```python
from build123d import *

# Parameters (mm, degrees)
SKETCH_1_R           = 3.5
EXTRUDE_1_DEPTH      = 3
SKETCH_2_R           = 1.5
CUT_EXTRUDE_1_DEPTH  = 10
EXTRUDE_2_DEPTH      = 4
EXTRUDE_5_DEPTH      = 7
FILLET_1_R           = 2
HOLE_WIZARD_M2_5_1_D = 2.05
SKETCH_12_R          = 1.025
EXTRUDE_6_DEPTH      = 5
EXTRUDE_7_DEPTH      = 2.5
CUT_EXTRUDE_START    = 2.5
SKETCH_14_W          = 65.294749478
SKETCH_14_H          = 102.548808998
CUT_EXTRUDE_2_DEPTH  = 93.634928881
CUT_EXTRUDE_3_DEPTH  = 2.5
SKETCH_16_R          = 1.35
CUT_EXTRUDE_4_DEPTH  = 10
EXTRUDE_START        = 1
SKETCH_17_R          = 1.35
EXTRUDE_8_DEPTH      = 1
FILLET_2_R           = 3


with BuildPart() as part:
    # 草图1 → 凸台-拉伸1 (new body)
    with BuildSketch(Plane.XY):
        with BuildLine():
            Line((0, 0), (17, 0))
            Line((17, 0), (17, 21))
            ThreePointArc((17, 21), (14.559389791, 26.961023013), (8.639106973, 29.498861644))
            ThreePointArc((8.639106973, 29.498861644), (4.214678609, 30.921411086), (1.327625741, 34.563407653))
            ThreePointArc((1.327625741, 34.563407653), (-5.234705957, 62.223549547), (-3.748501306, 90.612611571))
            ThreePointArc((-3.748501306, 90.612611571), (-5.162788524, 92.923505905), (-7.58241645, 91.704554856))
            ThreePointArc((-7.58241645, 91.704554856), (-12.196269834, 55.45091149), (0, 21))
            Line((0, 21), (0, 0))
        make_face()
        with Locations((8.5, 21)):
            Circle(SKETCH_1_R, mode=Mode.SUBTRACT)
    extrude(amount=EXTRUDE_1_DEPTH)

    # 草图2 → 切除-拉伸1 (cut)
    with BuildSketch(Plane(origin=(0, 0, 0), x_dir=(-1, 0, 0), z_dir=(0, 0, -1))):
        with Locations((-14, 4)):
            Circle(SKETCH_2_R)
        with Locations(Location((-3, 4, 0), (0, 0, 180))):
            Circle(SKETCH_2_R)
    extrude(amount=-CUT_EXTRUDE_1_DEPTH, mode=Mode.SUBTRACT)

    # 草图3 → 凸台-拉伸2 (add)
    with BuildSketch(Plane.XY.offset(3)):
        with BuildLine():
            ThreePointArc((-7.58241645, 91.704554856), (-12.6426678, 63.080202535), (-7.007767698, 34.563407653))
            Line((-7.007767698, 34.563407653), (1.327625741, 34.563407653))
            ThreePointArc((1.327625741, 34.563407653), (-5.234705957, 62.223549547), (-3.748501306, 90.612611571))
            ThreePointArc((-3.748501306, 90.612611571), (-5.162788524, 92.923505905), (-7.58241645, 91.704554856))
        make_face()
    extrude(amount=EXTRUDE_2_DEPTH)

    # 草图8 → 凸台-拉伸5 (add)
    with BuildSketch(Plane(origin=(0, 0, 0), x_dir=(-1, 0, 0), z_dir=(0, 0, -1))):
        with BuildLine():
            Line((8.353336216, 89.563407653), (13.622203114, 89.563407653))
            ThreePointArc((13.622203114, 89.563407653), (17.624786926, 61.957713987), (12.366747323, 34.563407653))
            Line((12.366747323, 34.563407653), (7.007767698, 34.563407653))
            ThreePointArc((7.007767698, 34.563407653), (12.623031035, 61.942490485), (8.353336216, 89.563407653))
        make_face()
    extrude(amount=-EXTRUDE_5_DEPTH)

    # 圆角1
    fillet_1_edges = [part.edges().sort_by_distance(p)[0] for p in [
        (-12.366747323, 34.563407653, 3.5),
        (-13.622203114, 89.563407653, 3.5),
        (-8.353336216, 89.563407653, 3.5),
        (-7.007767698, 34.563407653, 1.5),
    ]]
    fillet(fillet_1_edges, radius=FILLET_1_R)

    # M2.5 螺纹孔1 (through all)
    with Locations(Plane(origin=(0, 0, 0), x_dir=(-1, 0, 0), z_dir=(0, 0, -1))):
        with Locations((14.33753876, 52.418963936), (-20.3596947, 65.689324708), (13.008857265, 82.418963936), (15.069556912, 67.418963936)):
            Hole(HOLE_WIZARD_M2_5_1_D / 2)

    # 草图12 → 凸台-拉伸6 (add)
    with BuildSketch(Plane(origin=(0, 0, 0), x_dir=(-1, 0, 0), z_dir=(0, 0, -1))):
        with BuildLine():
            Line((7.545930127, 34.563407653), (8.350121818, 34.563407653))
            Line((8.350121818, 34.563407653), (10.964814809, 34.563407653))
            ThreePointArc((10.964814809, 34.563407653), (12.119748759, 34.930579564), (12.850623405, 35.897280083))
            ThreePointArc((12.850623405, 35.897280083), (17.623972952, 61.922380585), (14.065160369, 88.141182522))
            ThreePointArc((14.065160369, 88.141182522), (13.343005034, 89.168952691), (12.150434226, 89.563407653))
            Line((12.150434226, 89.563407653), (9.767172344, 89.563407653))
            Line((9.767172344, 89.563407653), (8.88187432, 89.563407653))
            ThreePointArc((8.88187432, 89.563407653), (13.123220294, 61.944160836), (7.545930127, 34.563407653))
        make_face()
        with Locations((14.33753876, 52.418963936)):
            Circle(SKETCH_12_R, mode=Mode.SUBTRACT)
        with Locations((15.069556912, 67.418963936)):
            Circle(SKETCH_12_R, mode=Mode.SUBTRACT)
        with Locations((13.008857265, 82.418963936)):
            Circle(SKETCH_12_R, mode=Mode.SUBTRACT)
    extrude(amount=EXTRUDE_6_DEPTH)

    # 草图13 → 凸台-拉伸7 (add)
    with BuildSketch(Plane(origin=(0, 0, -5), x_dir=(-1, 0, 0), z_dir=(0, 0, -1))):
        with BuildLine():
            Line((-1.327625741, 34.563407653), (7.545930127, 34.563407653))
            ThreePointArc((7.545930127, 34.563407653), (13.123220294, 61.944160836), (8.88187432, 89.563407653))
            Line((8.88187432, 89.563407653), (3.949832031, 89.563407653))
            ThreePointArc((3.949832031, 89.563407653), (5.185104579, 61.691682581), (-1.327625741, 34.563407653))
        make_face()
    extrude(amount=-EXTRUDE_7_DEPTH)

    # 草图14 → 切除-拉伸2 (cut, through all)
    with BuildSketch(Plane.XY.offset(-2.5).offset(CUT_EXTRUDE_START)):
        with Locations((4.683934874, 45.498546787)):
            Rectangle(SKETCH_14_W, SKETCH_14_H)
    extrude(amount=CUT_EXTRUDE_2_DEPTH, mode=Mode.SUBTRACT)

    # 草图15 → 切除-拉伸3 (cut)
    with BuildSketch(Plane.XY.offset(-2.5).offset(CUT_EXTRUDE_START)):
        with BuildLine():
            Line((-11.658303974, 48.563407653), (-16.239435818, 48.563407653))
            ThreePointArc((-16.239435818, 48.563407653), (-14.792540388, 42.164122556), (-12.850623405, 35.897280083))
            ThreePointArc((-12.850623405, 35.897280083), (-12.119748759, 34.930579564), (-10.964814809, 34.563407653))
            Line((-10.964814809, 34.563407653), (-7.545930127, 34.563407653))
            ThreePointArc((-7.545930127, 34.563407653), (-9.923992526, 41.468859633), (-11.658303974, 48.563407653))
        make_face()
    extrude(amount=-CUT_EXTRUDE_3_DEPTH, mode=Mode.SUBTRACT)

    # 草图16 → 切除-拉伸4 (cut)
    with BuildSketch(Plane.XY):
        with Locations((-13.008857265, 82.418963936)):
            Circle(SKETCH_16_R)
        with Locations((-15.069556912, 67.418963936)):
            Circle(SKETCH_16_R)
        with Locations((-14.33753876, 52.418963936)):
            Circle(SKETCH_16_R)
    extrude(amount=-CUT_EXTRUDE_4_DEPTH, mode=Mode.SUBTRACT)

    # 草图17 → 凸台-拉伸8 (add)
    with BuildSketch(Plane.XY.offset(EXTRUDE_START)):
        with BuildLine():
            Line((-16.239435818, 48.563407653), (-11.658303974, 48.563407653))
            ThreePointArc((-11.658303974, 48.563407653), (-12.965005338, 69.245901439), (-8.88187432, 89.563407653))
            Line((-8.88187432, 89.563407653), (-12.150434226, 89.563407653))
            ThreePointArc((-12.150434226, 89.563407653), (-13.343005034, 89.168952691), (-14.065160369, 88.141182522))
            ThreePointArc((-14.065160369, 88.141182522), (-17.520190498, 68.482379468), (-16.239435818, 48.563407653))
        make_face()
        with Locations((-14.33753876, 52.418963936)):
            Circle(SKETCH_17_R, mode=Mode.SUBTRACT)
        with Locations((-15.069556912, 67.418963936)):
            Circle(SKETCH_17_R, mode=Mode.SUBTRACT)
        with Locations((-13.008857265, 82.418963936)):
            Circle(SKETCH_17_R, mode=Mode.SUBTRACT)
    extrude(amount=-EXTRUDE_8_DEPTH)

    # 圆角2
    fillet_2_edges = [part.edges().sort_by_distance(p)[0] for p in [
        (-11.658303974, 48.563407653, -0.75),
    ]]
    fillet(fillet_2_edges, radius=FILLET_2_R)


solid = part.part
```
CAD build for the part. Positions are in the model's coordinates, mm. A direction names the side the tool comes from. Coordinates: 2 decimals unless noted, no trailing zeros. Order: outer loops, then holes, each group sorted by start corner. A loop starts at its lowest first (then second) coordinate and runs counter-clockwise, first axis right, second up.
(1) Saw through at A-A, the plane x = -5. Write the cut outline in (y, z), and give its area (3 significant figures).
Solution:
outline: (34.56, -5) - (59.93, -5) - (59.93, -2.5) - (34.56, -2.5) - close; (82.56, -5) - (89.56, -5) - (89.56, -2.5) - (82.56, -2.5) - close
area: 80.9 mm2
(2) Drill centre lines: L1, parallel to Z at x = -6, y = 66.5; L2, parallel to X at y = 65, z = -2.2; L3, parallel to X at y = 81.5, z = -1.65. Where is each one in solid material? Low to high.
Solution:
L1: z = -5 to -2.5
L2: x = -17.64 to -13.14
L3: x = -15.78 to -14, -12.02 to -11.17
(3) Pin check, flat tips, straight feed: pin 1 Ø1.5 at (x, y) = (-6.5, 54.5) entering from +Z; pin 2 Ø2 at (x, y) = (-3, 72) entering from -Z; pin 3 Ø1.1 at (x, z) = (-16, -0.5) entering from -Y. Stop position of each tip, or through.
Solution:
pin 1: stops at z = -2.5
pin 2: passes through
pin 3: stops at y = 48.56
(4) Which spindle directions (+Z, -Z, +X, -X, +Y, -Y) get a long thin tool onto all of the face, cutting with end or side? Do faces 5 (the face through (-16, 48.563, -1)), 6 (the face through (-14, 69, 1)). Say none if no direction does.
Solution:
face 5: +Z, +X, -X, -Y
face 6: +Z, +X, -X, +Y, -Y
(5) Saw through at C-C, the plane y = 56. Write the cut outline in (x, z), and give its area (3 significant figures).
Solution:
outline: (-17.28, -5) - (-4.47, -5) - (-4.47, -2.5) - (-12.76, -2.5) - (-12.76, 1) - (-17.28, 1) - close
area: 47.8 mm2
(6) Mould opens along X. For faces 1 (the face through (-15.245, 68.757, -1.958)), 2 (the face through (-12.106, 34.921, -3.732)), 3 (the face through (-5.22, 62.08, -3.77)), 4 (the face through (-14.513, 53.757, -1.958)) say: released by +X, released by -X, zero draft, split by the parting line, or undercut.
Solution:
face 1: undercut
face 2: released by -X
face 3: released by +X
face 4: undercut
(7) Saw through at D-D, the plane x = -7.75. Write the cut outline in (y, z).
Solution:
outline: (34.56, -5) - (89.56, -5) - (89.56, -2.5) - (34.56, -2.5) - close
(8) Saw through at B-B, the plane z = -0.8. Write the cut outline in (x, y).
Solution:
outline: (-16.24, 48.56) - (-15.22, 48.56) arc R3 ccw to (-12.26, 52.01) arc R79.5 cw to (-8.88, 89.56) - (-12.15, 89.56) arc R2 ccw to (-14.07, 88.14) arc R84 ccw to start; hole circle Ø2.7 at (-15.07, 67.42); hole circle Ø2.7 at (-14.34, 52.42); hole circle Ø2.7 at (-13.01, 82.42)
